```python
from build123d import *

# Parameters (mm, degrees)
F0_W     = 30
F0_H     = 1000
F1_DEPTH = 25
F2_W     = 6
F2_H     = 19
F3_DEPTH = 30.001
F4_DEPTH = 30.001
F5_W     = 200
F5_H     = 9.5
F5_W_2   = 194
F6_DEPTH = 4


with BuildPart() as f1:
    # F0 (on Top) → F1 (new body)
    with BuildSketch(Plane.XY):
        with Locations((-15, 500)):
            Rectangle(F0_W, F0_H)
    extrude(amount=F1_DEPTH)

    # F2 (on face) → F3 (cut, through all)
    with BuildSketch(Plane(origin=(-30, 0, 0), x_dir=(0, -1, 0), z_dir=(-1, 0, 0))):
        with Locations((-797, 15.5)):
            Rectangle(F2_W, F2_H)
    extrude(amount=-F3_DEPTH, mode=Mode.SUBTRACT)

    # F2 (on face) → F4 (cut, through all)
    with BuildSketch(Plane(origin=(-30, 0, 0), x_dir=(0, -1, 0), z_dir=(-1, 0, 0))):
        with Locations((-797, 15.5)):
            Rectangle(F2_W, F2_H)
        with Locations((-597, 15.5)):
            Rectangle(F2_W, F2_H)
        with Locations((-397, 15.5)):
            Rectangle(F2_W, F2_H)
        with Locations((-197, 15.5)):
            Rectangle(F2_W, F2_H)
    extrude(amount=-F4_DEPTH, mode=Mode.SUBTRACT)

    # F5 (on face) → F6 (cut)
    with BuildSketch(Plane(origin=(-30, 0, 0), x_dir=(0, -1, 0), z_dir=(-1, 0, 0))):
        with Locations((-900, 10.75)):
            Rectangle(F5_W, F5_H)
        with Locations((-697, 10.75)):
            Rectangle(F5_W_2, F5_H)
        with Locations((-297, 10.75)):
            Rectangle(F5_W_2, F5_H)
        with Locations((-497, 10.75)):
            Rectangle(F5_W_2, F5_H)
    extrude(amount=-F6_DEPTH, mode=Mode.SUBTRACT)


solid = f1.part
```
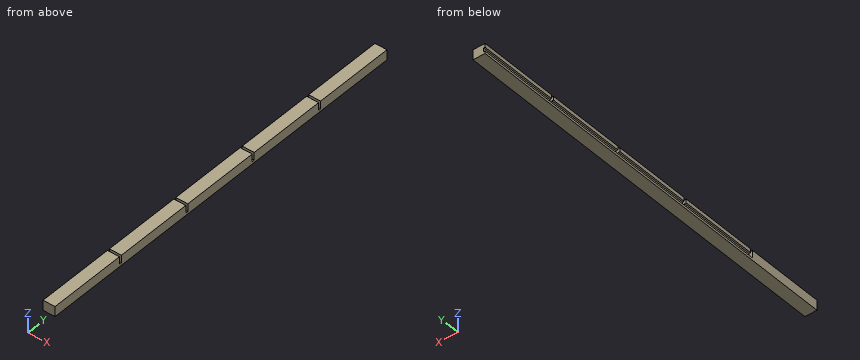
Read the model definition and answer for the solid it produces. Units are mm, in the model's axes. Coordinates: 2 decimals unless noted, no trailing zeros. Loops run counter-clockwise (first coordinate to the right, second up) from the corner with the lowest first, then second, coordinate; pieces in that order, holes last. Notation, with made-up numbers: (77.5, -40) -> (94.5, -40) arc R24 cw to (94.5, -17) -> close; hole circle Ø8 at (51, 84.5). An arc over 180 degrees is marked (long way). Return JSON: item names as keys, results as strings.
Item 1: Find the intervals of material crossed by probe 1 along Y at (x, z) = (-4.75, 22.5); probe 2 along X at (y, z) = (676, 7.25); probe 3 along Y at (x, z) = (-27, 12), in increasing order.
Answers:
{"probe 1": "y = 0 to 194, 200 to 394, 400 to 594, 600 to 794, 800 to 1000", "probe 2": "x = -26 to 0", "probe 3": "y = 0 to 194"}
Item 2: Find section B-B (y = 782.5). Determine the outline of the cut face in (x, z).
Answers:
{"outline": "(-30, 0) -> (0, 0) -> (0, 25) -> (-30, 25) -> (-30, 15.5) -> (-26, 15.5) -> (-26, 6) -> (-30, 6) -> close"}
Item 3: Find section C-C (x = -18). Determine the outline of the cut face in (y, z), plus the area to 3 significant figures.
Answers:
{"outline": "(0, 0) -> (1000, 0) -> (1000, 25) -> (800, 25) -> (800, 6) -> (794, 6) -> (794, 25) -> (600, 25) -> (600, 6) -> (594, 6) -> (594, 25) -> (400, 25) -> (400, 6) -> (394, 6) -> (394, 25) -> (200, 25) -> (200, 6) -> (194, 6) -> (194, 25) -> (0, 25) -> close", "area": "24,500 mm2"}
Item 4: Find section A-A (z = 19.5). Determine the outline of the cut face in (x, y), plus the area to 3 significant figures.
Answers:
{"outline": "(-30, 0) -> (0, 0) -> (0, 194) -> (-30, 194) -> close; (-30, 200) -> (0, 200) -> (0, 394) -> (-30, 394) -> close; (-30, 400) -> (0, 400) -> (0, 594) -> (-30, 594) -> close; (-30, 600) -> (0, 600) -> (0, 794) -> (-30, 794) -> close; (-30, 800) -> (0, 800) -> (0, 1000) -> (-30, 1000) -> close", "area": "29,300 mm2"}
Item 5: A flat-ended cylindrical pin translates along its axis: P1, Ø5, axis at y = 358.5, z = 10.5, coming from the -X side. Find the tip coordinate at first contact, or state that the pin passes through.
Answers:
{"P1": "stops at x = -26"}
